```python
from build123d import *

# Parameters (mm, degrees)
F0_W     = 121
F0_H     = 16
F1_DEPTH = 57
F2_R     = 7
F3_DEPTH = 16.001
F4_DEPTH = 38
F5_DEPTH = 38
F7_DEPTH = 57.001


with BuildPart() as f1:
    # F0 (on Top) → F1 (new body)
    with BuildSketch(Plane.XY):
        with Locations((0, 8)):
            Rectangle(F0_W, F0_H)
    extrude(amount=F1_DEPTH)

    # F2 (on face) → F3 (cut, through all)
    with BuildSketch(Plane.XZ):
        with Locations((-16.5, 41)):
            Circle(F2_R)
        with Locations((16.5, 12)):
            Circle(F2_R)
    extrude(amount=-F3_DEPTH, mode=Mode.SUBTRACT)

    # F2 (on face) → F4 (join)
    with BuildSketch(Plane.XZ):
        Polygon((-60.5, 46), (-60.5, 0), (-38.5, 0), (-38.5, 29.272727), align=None)
        Polygon((-38.5, 29.272727), (-38.5, 0), (0, 0), align=None)
    extrude(amount=F4_DEPTH)

    # F2 (on face) → F5 (join)
    with BuildSketch(Plane.XZ):
        Polygon((60.5, 57), (1.5, 57), (60.5, 11), align=None)
    extrude(amount=F5_DEPTH)

    # F6 (on face) → F7 (cut, through all)
    with BuildSketch(Plane.XY.offset(57)):
        Polygon((0, -25.555556), (-38.5, -38), (0, -38), align=None)
        Polygon((60.5, -6), (1.5, -25.070707), (1.5, -38), (60.5, -38), align=None)
    extrude(amount=-F7_DEPTH, mode=Mode.SUBTRACT)


solid = f1.part
```
Geometry: final body of the model. Coordinates: model frame, mm. A direction names the side the tool comes from. Round coordinates to 2 decimals unless told otherwise and drop trailing zeros. Write each loop counter-clockwise with the first axis right and the second up, starting at its lowest first coordinate (ties: lowest second). Pieces come first, ordered by that corner, then holes. Notation, with made-up numbers: (6, 72) -> (53, 72) arc R13 cw to (53, 82) -> close; hole circle Ø2 at (66, 8). An arc over 180 degrees is marked (long way). Return JSON: item names as keys, results as strings.
Q1. Section D-D on z = 9.5. Return the cut outline in (x, y).
From the geometry:
{"outline": "(-60.5, -38) -> (-38.5, -38) -> (-12.49, -29.59) -> (-12.49, 0) -> (9.96, 0) -> (9.96, 16) -> (-60.5, 16) -> close; (23.04, 0) -> (60.5, 0) -> (60.5, 16) -> (23.04, 16) -> close"}
Q2. Section C-C on x = 16.5. Return the cut outline in (y, z), and give its area (3 significant figures).
From the geometry:
{"outline": "(-20.22, 45.31) -> (0, 45.31) -> (0, 19) -> (16, 19) -> (16, 57) -> (-20.22, 57) -> close; (0, 0) -> (16, 0) -> (16, 5) -> (0, 5) -> close", "area": "924 mm2"}
Q3. Ray query, line 1 (Z direction, x = 16.5, y = 5.75); line 2 (Z direction, x = -16, y = 8); line 3 (Y direction, x = 0, z = 15). Return the intervals inside material, ascending.
From the geometry:
{"line 1": "0 to 5, 19 to 57", "line 2": "0 to 34.02, 47.98 to 57", "line 3": "0 to 16"}
Q4. Section A-A on y = 4. Return the cut outline in (x, z), and give its area (3 significant figures).
From the geometry:
{"outline": "(-60.5, 0) -> (60.5, 0) -> (60.5, 57) -> (-60.5, 57) -> close; hole circle Ø14 at (-16.5, 41); hole circle Ø14 at (16.5, 12)", "area": "6,590 mm2"}
Q5. First-contact query: pin 1 Ø8.5 at (x, z) = (-16.5, 41) entering from -Y; pin 2 Ø1 at (x, z) = (-15.5, 34) entering from -Y; pin 3 Ø2 at (x, z) = (14, 48.5) entering from -Y; pin 4 Ø1 at (x, y) = (-20.5, -7) entering from +Z. Flat tips, straight axial feed; report the tip coordinate or a pass-through.
From the geometry:
{"pin 1": "through", "pin 2": "y = 0", "pin 3": "y = -21.35", "pin 4": "z = 15.97"}
Q6. Section B-B on z = 36.5. Return the cut outline in (x, y), and give its area (3 significant figures).
From the geometry:
{"outline": "(-60.5, -38) -> (-48.01, -38) -> (-48.01, 0) -> (-21.86, 0) -> (-21.86, 16) -> (-60.5, 16) -> close; (-11.14, 0) -> (27.79, 0) -> (27.79, -16.57) -> (60.5, -6) -> (60.5, 16) -> (-11.14, 16) -> close", "area": "2,610 mm2"}
Q7. Mould query, pull axis Z, two halves, no side actions, for faces 1 (the flat face through (-1, 16, 28)), 2 (the cylindrical face through (9.507, 7.888, 12.308)), 3 (the flat face through (-14, -5, 0)), 4 (the cylindrical face through (-21.66, 7.89, 45.73)). Classes: +Z half, -Z half, draft (parallel to the pull), parting line (faces both ways), or undercut.
From the geometry:
{"face 1": "draft", "face 2": "undercut", "face 3": "-Z half", "face 4": "undercut"}
Q8. Set-up query: faces 5 (the flat face through (60.5, 5, 28)), 6 (the flat face through (24.031, -9.574, 39.433)), 7 (the flat face through (-1, 0, 28)). Return all of +Z, -Z, +X, -X, +Y, -Y with unobstructed straight access to the full face (end or side cutting, diameter ignored); none if empty.
From the geometry:
{"face 5": "+Z, -Z, +X, +Y, -Y", "face 6": "-Z, -Y", "face 7": "-Y"}
